Geometry: final body of the model. Coordinates: model frame, mm. A direction names the side the tool comes from. Round coordinates to 2 decimals unless told otherwise and drop trailing zeros. Write each loop counter-clockwise with the first axis right and the second up, starting at its lowest first coordinate (ties: lowest second). Pieces come first, ordered by that corner, then holes. Notation, with made-up numbers: (20.25, 80) - (74.25, 80) arc R19 ccw to (74.25, 107) - close; hole circle Ø5 at (66, -11.5). An arc over 180 degrees is marked (long way). Use a Markdown table: item, result. Add a question column.
```python
from build123d import *

# Parameters (mm, degrees)
F1_DEPTH = 20
F2_W     = 20
F2_H     = 20
F3_DEPTH = 26.001
F5_DEPTH = 40.001


with BuildPart() as f1:
    # F0 (on Top) → F1 (new body, symmetric)
    with BuildSketch(Plane.XY):
        Polygon((0, 26), (0, 0), (10, 0), (10, 13), (50, 13), (50, 39), (40, 39), (40, 26), align=None)
    extrude(amount=F1_DEPTH, both=True)

    # F2 (on face) → F3 (cut, through all)
    with BuildSketch(Plane.XZ.offset(-13)):
        with Locations((40, 0)):
            Rectangle(F2_W, F2_H)
    extrude(amount=-F3_DEPTH, mode=Mode.SUBTRACT)

    # F4 (on face) → F5 (cut, through all)
    with BuildSketch(Plane.XY.offset(20)):
        Polygon((0, 0), (10, 26), (0, 26), align=None)
    extrude(amount=-F5_DEPTH, mode=Mode.SUBTRACT)


solid = f1.part
```
1) Section D-D, the plane y = 18. Return the cut outline in (x, z).
2) Pin query (flat end, axial travel): P1, Ø6, axis at x = 13.5, z = 5.5, coming from the +Y side; P2, Ø5, axis at y = 30.5, z = -15.5, coming from the -X side; P3, Ø10.5, axis at y = 7, z = -3, coming from the +X side. Return the tip coordinate at first contact, or that it passes through.
3) Section B-B, the plane y = 28.5. Return the cut outline in (x, z).
4) Section A-A, the plane x = 42. Return the cut outline in (y, z).
5) Section C-C, the plane z = 0. Return the cut outline in (x, y), then the cut area to 3 significant figures.
6) Draft query along Z for faces 6 (the flat face through (30, 19, 0)), 7 (the flat face through (30, 20, 20)), 8 (the flat face through (50, 26, -15)), 9 (the flat face through (42, 23, -10)). Return one class per face: released by +Z, released by -Z, zero draft, split by the parting line, or undercut.
7) Material intervals for L1, parallel to Z at x = 45, y = 32.5; L2, parallel to Y at x = 29.5, z = 5; L3, parallel to Y at x = 46.5, z = -13, sorted ascending. Write a range as from..to.
8) Set-up query: faces 1 (the flat face through (50, 26, 15)), 2 (the flat face through (22, 26, 0)), 3 (the flat face through (25, 13, 0)), 4 (the flat face through (5, 0, 0)), 5 (the flat face through (42, 23, 10)). Return all of +Z, -Z, +X, -X, +Y, -Y with unobstructed straight access to the full face (end or side cutting, diameter ignored); none if empty.
Output values:
| question | item | result |
|---|---|---|
| 1 | outline | (6.92, -20) - (50, -20) - (50, -10) - (30, -10) - (30, 10) - (50, 10) - (50, 20) - (6.92, 20) - close |
| 2 | P1 | stops at y = 26 |
| 2 | P2 | stops at x = 40 |
| 2 | P3 | stops at x = 10 |
| 3 | outline | (40, -20) - (50, -20) - (50, -10) - (40, -10) - close; (40, 10) - (50, 10) - (50, 20) - (40, 20) - close |
| 4 | outline | (13, -20) - (39, -20) - (39, -10) - (13, -10) - close; (13, 10) - (39, 10) - (39, 20) - (13, 20) - close |
| 5 | outline | (0, 0) - (10, 0) - (10, 13) - (30, 13) - (30, 26) - (10, 26) - close |
| 5 | area | 390 mm^2 |
| 6 | face 6 | undercut |
| 6 | face 7 | released by +Z |
| 6 | face 8 | zero draft |
| 6 | face 9 | undercut |
| 7 | L1 | z = -20..-10, 10..20 |
| 7 | L2 | y = 13..26 |
| 7 | L3 | y = 13..39 |
| 8 | face 1 | +Z, -Z, +X, +Y, -Y |
| 8 | face 2 | +Z, -Z, -X, +Y |
| 8 | face 3 | +Z, -Z, +X, -Y |
| 8 | face 4 | +Z, -Z, +X, -X, -Y |
| 8 | face 5 | +X, +Y, -Y |
